from build123d import *

# Parameters (mm, degrees)
BOSS_EXTRU_1_DEPTH      = 30
ESQUISSE2_R             = 2.5
ENL_V_MAT_EXTRU_1_DEPTH = 54.945473789
ESQUISSE4_R             = 4.5
ENL_V_MAT_EXTRU_2_DEPTH = 57.869272391


with BuildPart() as part:
    # Esquisse1 → Boss.-Extru.1 (new body)
    with BuildSketch(Plane(origin=(0, 0, 0), x_dir=(0, 0, -1), z_dir=(1, 0, 0))):
        Polygon((0, 0), (33.318375445, -30), (-8.893874852, -30), (-20, -20), (0, -20), align=None)
    extrude(amount=BOSS_EXTRU_1_DEPTH)

    # Esquisse2 → Enlèv. mat.-Extru.1 (cut, through all)
    with BuildSketch(Plane(origin=(0, 0, 0), x_dir=(1, 0, 0), z_dir=(0, 0.7431448254773982, -0.6691306063588538))):
        with Locations(Location((15, 17.867207619, 0), (0, 0, 270))):
            Circle(ESQUISSE2_R)
    extrude(amount=-ENL_V_MAT_EXTRU_1_DEPTH, mode=Mode.SUBTRACT)

    # Esquisse4 → Enlèv. mat.-Extru.2 (cut, through all)
    with BuildSketch(Plane(origin=(0, -13.376606859, 12.044350914), x_dir=(1, 0, 0), z_dir=(0, 0.7431448254773982, -0.6691306063588538))):
        with Locations(Location((15, 17.867207619, 0), (0, 0, 270))):
            Circle(ESQUISSE4_R)
    extrude(amount=-ENL_V_MAT_EXTRU_2_DEPTH, mode=Mode.SUBTRACT)


solid = part.part
Design review of the part built by this model. Coordinates are the model's own, in mm. A direction names the side the tool comes from. Round coordinates to 2 decimals unless told otherwise and drop trailing zeros. Write each loop counter-clockwise with the first axis right and the second up, starting at its lowest first coordinate (ties: lowest second). Pieces come first, ordered by that corner, then holes. Notation, with made-up numbers: (70, 71) -> (117, 71) arc R34 ccw to (117, 106) -> close; hole circle Ø7 at (28, -24.75). An arc over 180 degrees is marked (long way). One line per question, with ' | ' between items.
(1) Take a section at D-D, the plane z = -29. State the section outline as (x, y) points.
Result sheet:
outline: (0, -30) -> (30, -30) -> (30, -26.11) -> (0, -26.11) -> close
(2) Machinability: for faces 5 (the cylindrical face through (14.042, -17.005, -5.624)), 6 (the flat face through (15, -10, 0)), which of the approach directions +Z, -Z, +X, -X, +Y, -Y give a long, thin tool a straight path to every point of the face, cutting with its end or side? Answer none if there is none.
Result sheet:
face 5: none | face 6: +Z, +X, -X, +Y
(3) Insertion check: P1, Ø3, axis at x = 17, y = -15.5, coming from the +Z side; P2, Ø1, axis at x = 6.5, z = 12.5, coming from the -Y side; P3, Ø1, axis at x = 9.5, z = -2.5, coming from the +Y side. Each pin has a flat end and moves straight along its axis. Give the tip position at first contact, or say it passes through.
Result sheet:
P1: z = 0 | P2: y = -27.2 | P3: y = -1.8
(4) Take a section at C-C, the plane y = -1.5. State the section outline as (x, z) points.
Result sheet:
outline: (0, -1.67) -> (30, -1.67) -> (30, 0) -> (0, 0) -> close
(5) Draft analysis for pull direction X (two halves, no side actions). For faces 1 (the flat face through (30, -21, -7)), 2 (the flat face through (13.063, -24.036, 0.206)), 3 (the cylindrical face through (16.352, -25.368, 4.574)), 4 (the flat face through (14.79, -25.07, 14.37)), state which applies: released by +X, released by -X, zero draft, split by the parting line, or undercut.
Result sheet:
face 1: released by +X | face 2: undercut | face 3: undercut | face 4: zero draft
(6) Take a section at A-A, the plane x = 8.5. State the section outline as (y, z) points, and give its area (3 significant figures).
Result sheet:
outline: (-30, -33.32) -> (0, 0) -> (-20, 0) -> (-20, 20) -> (-30, 8.89) -> close | area: 644 mm2
(7) Wall thickness on line 1 (X direction, y = -28.5, z = 2.5); line 2 (Y direction, x = 15.5, z = -11); line 3 (Y direction, x = 25.5, z = 6.5): over which ranges is each line inside the solid? List them lowest first. Write a range as [from, to].
Result sheet:
line 1: [0, 10.55], [19.45, 30] | line 2: [-30, -18.15], [-10.82, -9.9] | line 3: [-30, -20]
(8) Take a section at B-B, the plane z = -4. State how many separate pieces and enclosed holes the cut face has, and give its area (3 significant figures).
Result sheet:
separate pieces: 1 | enclosed holes: 2 | area: 759 mm2
